Source: CAD feature listing. Evaluate the final solid. Frame: model axes, mm. Round coordinates to 2 decimals unless told otherwise and drop trailing zeros. Loops run counter-clockwise (first coordinate to the right, second up) from the corner with the lowest first, then second, coordinate; pieces in that order, holes last. Notation, with made-up numbers: (47.5, 34.25) - (103.5, 34.25) arc R29 cw to (103.5, 71.25) - close; hole circle Ø11 at (21, 29). An arc over 180 degrees is marked (long way). One line per question, with ' | ' between items.
from build123d import *

# Parameters (mm, degrees)
SKETCH1_W           = 100
SKETCH1_H           = 100
SKETCH1_R           = 2.5
SKETCH1_R_2         = 2.25
BOSS_EXTRUDE1_DEPTH = 0.8
SKETCH2_R           = 44.3
CUT_EXTRUDE1_DEPTH  = 71.728777736


with BuildPart() as part:
    # Sketch1 → Boss-Extrude1 (new, symmetric)
    with BuildSketch(Plane(origin=(0, 0, 0), x_dir=(1, 0, 0), z_dir=(0, 1, 0))):
        Rectangle(SKETCH1_W, SKETCH1_H)
        with Locations(Location((-40, -40, 0), (0, 0, 270))):
            Circle(SKETCH1_R, mode=Mode.SUBTRACT)
        with Locations(Location((-40, -20, 0), (0, 0, 270))):
            Circle(SKETCH1_R, mode=Mode.SUBTRACT)
        with Locations(Location((40, -20, 0), (0, 0, 270))):
            Circle(SKETCH1_R, mode=Mode.SUBTRACT)
        with Locations(Location((-41.2, 41.2, 0), (0, 0, 270))):
            Circle(SKETCH1_R_2, mode=Mode.SUBTRACT)
        with Locations(Location((41.2, 41.2, 0), (0, 0, 270))):
            Circle(SKETCH1_R_2, mode=Mode.SUBTRACT)
    extrude(amount=BOSS_EXTRUDE1_DEPTH, both=True)

    # Sketch2 → Cut-Extrude1 (cut, through all)
    with BuildSketch(Plane(origin=(0, 0.8, 0), x_dir=(1, 0, 0), z_dir=(0, 1, 0))):
        with Locations((0, 82.44)):
            Circle(SKETCH2_R)
    extrude(amount=-CUT_EXTRUDE1_DEPTH, mode=Mode.SUBTRACT)


solid = part.part
1. Section query D-D, the plane x = 41.2. Return loops of the section in (y, z), plus the area to 3 significant figures.
Worked out:
outline: (-0.8, -50) - (0.8, -50) - (0.8, -43.45) - (-0.8, -43.45) - close; (-0.8, -38.95) - (0.8, -38.95) - (0.8, 17.81) - (-0.8, 17.81) - close; (-0.8, 22.19) - (0.8, 22.19) - (0.8, 50) - (-0.8, 50) - close | area: 146 mm2
2. Section query A-A, the plane z = 20. Return loops of the section in (x, y).
Worked out:
outline: (-50, -0.8) - (-42.5, -0.8) - (-42.5, 0.8) - (-50, 0.8) - close; (-37.5, -0.8) - (37.5, -0.8) - (37.5, 0.8) - (-37.5, 0.8) - close; (42.5, -0.8) - (50, -0.8) - (50, 0.8) - (42.5, 0.8) - close
3. Material intervals for probe 1 along X at (y, z) = (0.4, 20); probe 2 along X at (y, z) = (-0.6, 40); probe 3 along Z at (x, y) = (-38.5, 0.1), sorted ascending.
Worked out:
probe 1: x = -50 to -42.5, -37.5 to 37.5, 42.5 to 50 | probe 2: x = -50 to -42.5, -37.5 to 50 | probe 3: z = -50 to 18, 22 to 38, 42 to 50
4. Mould query, pull axis Z, two halves, no side actions, for faces 1 (the flat face through (-1, -0.8, -1)), 2 (the cylindrical face through (-0.465, 0.011, -38.142)), 3 (the cylindrical face through (-40.96, -0.01, 42.31)). Classes: released by +Z, released by -Z, zero draft, split by the parting line, or undercut.
Worked out:
face 1: zero draft | face 2: released by -Z | face 3: undercut
5. Section query C-C, the plane y = -0.3. Return loops of the section in (x, z).
Worked out:
outline: (-50, -50) - (-30.17, -50) arc R44.3 cw to (30.17, -50) - (50, -50) - (50, 50) - (-50, 50) - close; hole circle Ø4.5 at (-41.2, -41.2); hole circle Ø5 at (-40, 20); hole circle Ø5 at (-40, 40); hole circle Ø5 at (40, 20); hole circle Ø4.5 at (41.2, -41.2)
6. Section query B-B, the plane x = -41.2. Return loops of the section in (y, z).
Worked out:
outline: (-0.8, -50) - (0.8, -50) - (0.8, -43.45) - (-0.8, -43.45) - close; (-0.8, -38.95) - (0.8, -38.95) - (0.8, 17.81) - (-0.8, 17.81) - close; (-0.8, 22.19) - (0.8, 22.19) - (0.8, 37.81) - (-0.8, 37.81) - close; (-0.8, 42.19) - (0.8, 42.19) - (0.8, 50) - (-0.8, 50) - close
7. Contact query for flat-ended pins moving along their axis: P1, Ø3.5, axis at x = -41.2, z = -41.2, coming from the +Y side; P2, Ø6.5, axis at x = -40, z = 40, coming from the -Y side. Output: stop coordinate, or through.
Worked out:
P1: passes through | P2: stops at y = -0.8
